CAD build for the part. Positions are in the model's coordinates, mm. A direction names the side the tool comes from. Coordinates: 2 decimals unless noted, no trailing zeros. Write each loop counter-clockwise with the first axis right and the second up, starting at its lowest first coordinate (ties: lowest second). Pieces come first, ordered by that corner, then holes.
```python
from build123d import *

# Parameters (mm, degrees)
F0_R          = 38
F0_R_2        = 26.5
F1_DEPTH      = 18
F1_DEPTH_BACK = 4
F3_DEPTH      = 5.4
F5_DEPTH      = 16.601
F7_D          = 5
F8_D          = 20


with BuildPart() as f1:
    # F0 (on Top) → F1 (new body, two sides)
    with BuildSketch(Plane.XY) as f1_sk:
        Circle(F0_R)
        Circle(F0_R_2, mode=Mode.SUBTRACT)
    extrude(amount=F1_DEPTH)
    extrude(f1_sk.sketch, amount=-F1_DEPTH_BACK)

    # F2 (on face) → F3 (join)
    with BuildSketch(Plane.XY.offset(18)):
        with BuildLine():
            Line((-35.327043, 14), (-40.657103, 14))
            ThreePointArc((-40.657103, 14), (-43, 0), (-40.657103, -14))
            Line((-40.657103, -14), (-35.327043, -14))
            ThreePointArc((-35.327043, -14), (-38, 0), (-35.327043, 14))
        make_face()
        with BuildLine():
            Line((-28.217902, 14), (-35.327043, 14))
            ThreePointArc((-35.327043, 14), (-38, 0), (-35.327043, -14))
            Line((-35.327043, -14), (-28.217902, -14))
            ThreePointArc((-28.217902, -14), (-31.5, 0), (-28.217902, 14))
        make_face()
        with BuildLine():
            ThreePointArc((38, 0), (37.32578, 7.126442), (35.327043, 14))
            Line((35.327043, 14), (28.217902, 14))
            ThreePointArc((28.217902, 14), (31.5, 0), (28.217902, -14))
            Line((28.217902, -14), (35.327043, -14))
            ThreePointArc((35.327043, -14), (37.32578, -7.126442), (38, 0))
        make_face()
        with BuildLine():
            Line((40.657103, 14), (35.327043, 14))
            ThreePointArc((35.327043, 14), (37.32578, 7.126442), (38, 0))
            ThreePointArc((38, 0), (37.32578, -7.126442), (35.327043, -14))
            Line((35.327043, -14), (40.657103, -14))
            ThreePointArc((40.657103, -14), (43, 0), (40.657103, 14))
        make_face()
    extrude(amount=-F3_DEPTH)

    # F4 (on face) → F5 (cut, through all)
    with BuildSketch(Plane(origin=(0, 0, 12.6), x_dir=(1, 0, 0), z_dir=(0, 0, -1))):
        with BuildLine():
            Line((-15.099669, 16), (-34.467376, 16))
            ThreePointArc((-34.467376, 16), (-38, 0), (-34.467376, -16))
            Line((-34.467376, -16), (-15.099669, -16))
            ThreePointArc((-15.099669, -16), (-22, 0), (-15.099669, 16))
        make_face()
        with BuildLine():
            ThreePointArc((15.099669, 16), (22, 0), (15.099669, -16))
            Line((15.099669, -16), (34.467376, -16))
            ThreePointArc((34.467376, -16), (38, 0), (34.467376, 16))
            Line((34.467376, 16), (15.099669, 16))
        make_face()
    extrude(amount=F5_DEPTH, mode=Mode.SUBTRACT)

    # F7 (through all)
    with Locations(Plane.XY.offset(18)):
        with Locations((-37, 0), (37, 0)):
            Hole(F7_D / 2)

    # F8 (through all)
    with Locations(Plane.XY.offset(18)):
        with Locations((-29.304576, 27.955175), (29.304576, -27.955175)):
            Hole(F8_D / 2)


solid = f1.part
```
Item 1: Saw through at B-B, the plane y = 0. Write the cut outline in (x, z), and give its area (3 significant figures).
Item 2: Which spindle directions (+Z, -Z, +X, -X, +Y, -Y) get a long thin tool onto all of the face, cutting with end or side? Do faces 1 (the flat face through (-32, 0, 12.6)), 2 (the flat face through (-38, -14, 15)), 3 (the flat face through (-10, 26, 18)), 4 (the cylindrical face through (-21.954, 21.175, 6.846)), 5 (the flat face through (38, -14, 15)). Say none if no direction does.
Item 3: Flat gauge pins, fed straight in: pin 1 Ø4.5 at (x, z) = (39, 14.5) entering from +Y; pin 2 Ø4 at (x, z) = (25.5, 11.5) entering from -Y; pin 3 Ø10.5 at (x, z) = (-28, 1.5) entering from +Y. Where does each tip first touch, or does it go through?
Item 4: Saw through at A-A, the plane x = 0. Write the cut outline in (y, z), and give its area (3 significant figures).
Item 5: Wall check: line 1 along Y through (x, z) = (37, 13.85); line 2 along Y through (x, z) = (0, 13.25); line 3 along X through (y, z) = (-24, 12.75). Give the ranges that are in metal, low to high.
Item 6: Two-plate mould, pull along X, no slides. Class faces 6 (the flat face through (0, -27, -4)), 7 (the cylindrical face through (-34.015, 16.94, 9.598)), 8 (the cylindrical face through (34.69, -0.96, 15.26)): +X half, -X half, draft (parallel to the pull), parting line (faces both ways), or undercut.
Item 7: Saw through at C-C, the plane z = 11.25. Write the cut outline in (x, y).
Item 8: Saw through at D-D, the plane y = 21. Write the cut outline in (x, z).
Working result:
1. outline: (-43, 12.6) - (-39.5, 12.6) - (-39.5, 18) - (-43, 18) - close; (-34.5, 12.6) - (-26.5, 12.6) - (-26.5, 18) - (-34.5, 18) - close; (26.5, 12.6) - (34.5, 12.6) - (34.5, 18) - (26.5, 18) - close; (39.5, 12.6) - (43, 12.6) - (43, 18) - (39.5, 18) - close
1. area: 124 mm2
2. face 1: -Z, +X, -X
2. face 2: +Z, -Z, -X, -Y
2. face 3: +Z, +X, -X, +Y, -Y
2. face 4: +Z, -Z
2. face 5: +Z, -Z, +X, -Y
3. pin 1: stops at y = 14
3. pin 2: stops at y = -19.81
3. pin 3: stops at y = 20.4
4. outline: (-38, -4) - (-26.5, -4) - (-26.5, 18) - (-38, 18) - close; (26.5, -4) - (38, -4) - (38, 18) - (26.5, 18) - close
4. area: 506 mm2
5. line 1: y = -14 to -2.5, 2.5 to 14
5. line 2: y = -38 to -26.5, 26.5 to 38
5. line 3: x = -29.46 to -11.24, 11.24 to 20.12
6. face 6: draft
6. face 7: -X half
6. face 8: undercut
7. outline: (-34.47, -16) arc R38 ccw to (20.23, -32.17) arc R10 cw to (33.08, -18.7) arc R38 ccw to (34.47, -16) - (21.12, -16) arc R26.5 cw to (-21.12, -16) - close; (-34.47, 16) - (-21.12, 16) arc R26.5 cw to (21.12, 16) - (34.47, 16) arc R38 ccw to (-20.23, 32.17) arc R10 cw to (-33.08, 18.7) arc R38 ccw to start
8. outline: (-22.12, -4) - (-16.16, -4) - (-16.16, 18) - (-22.12, 18) - close; (16.16, -4) - (31.67, -4) - (31.67, 18) - (16.16, 18) - close
